from build123d import *

# Parameters (mm, degrees)
BOSS_EXTRUDE1_DEPTH = 6
SKETCH2_R           = 0.5
BOSS_EXTRUDE2_DEPTH = 6


with BuildPart() as part:
    # Sketch1 → Boss-Extrude1 (new body)
    with BuildSketch(Plane(origin=(0, 0, 0), x_dir=(1, 0, 0), z_dir=(0, 1, 0))):
        Polygon((5.804365786, 4.796692747), (5.804365786, 10.796692747), (5.804365786, 18.796692747), (18.804365786, 18.796692747), (25, 18.796692747), (40, 18.796692747), (40, 48.796692747), (25, 48.796692747), (25, 103.796692747), (0, 103.796692747), (0, 144.796692747), (200, 144.796692747), (200, 4.796692747), align=None)
    extrude(amount=BOSS_EXTRUDE1_DEPTH)

    # Sketch2 → Boss-Extrude2 (add)
    with BuildSketch(Plane.XY.offset(-4.796692747)):
        with BuildLine():
            Line((7.804365786, 6), (17.804365786, 6))
            Line((17.804365786, 6), (17.804365786, 11))
            ThreePointArc((17.804365786, 11), (12.804365786, 16), (7.804365786, 11))
            Line((7.804365786, 11), (7.804365786, 6))
        make_face()
        with Locations((12.804365786, 11)):
            Circle(SKETCH2_R, mode=Mode.SUBTRACT)
    extrude(amount=-BOSS_EXTRUDE2_DEPTH)


solid = part.part
Verification items for the finished model (mm, model axes). A direction names the side the tool comes from. Coordinates: 2 decimals unless noted, no trailing zeros. Order: outer loops, then holes, each group sorted by start corner. A loop starts at its lowest first (then second) coordinate and runs counter-clockwise, first axis right, second up. Notation, with made-up numbers: M 69.25,85.5 L 97.25,85.5 A20 ccw 97.25,119.5 Z; hole C -2,37.25 d3. An arc over 180 degrees is marked long. One line per item, written item: value. Start each with the question number.
Item 1: Sectioned sample at A-A (z = -93.5). Enter the section's corners in (x, y), then the cut area to 3 significant figures.
Item 2: Scan lines: probe 1 along X at (y, z) = (1.25, -90); probe 2 along Y at (x, z) = (147.5, -61); probe 3 along X at (y, z) = (3.5, -39). Record each from-to range of solid material in increasing order.
Item 3: Gauge pin test, flat ends, axial feed: pin 1 (3 mm diameter, centred on y = 3, z = -74, fed in from -X); pin 2 (4 mm diameter, centred on x = 135.5, z = -68.5, fed in from +Y); pin 3 (1.8 mm diameter, centred on y = 3, z = -28.5, fed in from -X). Record the tip position at first contact, or that the pin passes through.
Item 4: Sectioned sample at B-B (x = 109). Enter the section's corners in (y, z), then the cut area to 3 significant figures.
Item 5: Access from +Z, -Z, +X, -X, +Y, -Y to the whole of each face (thin tool, end or side, straight path). Record for faces 1 (the flat face through (7.804, 9, -8)), 2 (the flat face through (17.804, 8, -8)), 3 (the flat face through (13, 10, -10.797)), 4 (the flat face through (40, 3, -34)), 5 (the flat face through (5.804, 3, -12)).
Item 6: Mould release check, pull along Z, two halves, no side actions. Record for faces 6 (the flat face through (99, 3, -144.797)), 7 (the flat face through (13, 3, -103.797)), 8 (the flat face through (96, 4, -4.797)): released by +Z, released by -Z, zero draft, split by the parting line, or undercut.
Conclusion:
1. outline: M 25,0 L 200,0 L 200,6 L 25,6 Z
1. area: 1,050 mm^2
2. probe 1: x = 25 to 200
2. probe 2: y = 0 to 6
2. probe 3: x = 40 to 200
3. pin 1: stops at x = 25
3. pin 2: stops at y = 6
3. pin 3: stops at x = 40
4. outline: M 0,-144.8 L 6,-144.8 L 6,-4.8 L 0,-4.8 Z
4. area: 840 mm^2
5. face 1: +Z, -Z, -X, +Y
5. face 2: +Z, -Z, +X, +Y
5. face 3: -Z, +X, -X, +Y
5. face 4: -X, +Y, -Y
5. face 5: +Z, -X, +Y, -Y
6. face 6: released by -Z
6. face 7: undercut
6. face 8: released by +Z
